from build123d import *

# Parameters (mm, degrees)
F1_DEPTH = 12.7


with BuildPart() as f1:
    # F0 (on Top) → F1 (new body)
    with BuildSketch(Plane.XY):
        with BuildLine():
            Line((0, 52.0365796983), (-20.0025, 52.0365796983))
            Line((-20.0025, 52.0365796983), (-12.633157894, -20.4536858946))
            Line((-12.633157894, -20.4536858946), (-20.0025, -42.7121035755))
            add(Edge.make_bspline(
                [(-20.0025, -42.7121035755), (-21.1866346696, -45.1468080489), (-23.1579199792, -48.7548194432), (-25.0683852323, -64.3099806953), (-16.9383073123, -59.2079587227), (-13.8363149017, -62.2634203017)],
                knots=[0, 0, 0, 0, 0.3090403224, 0.6689788708, 1, 1, 1, 1], degree=3))
            Line((-13.8363149017, -62.2634203017), (0, -62.2634203017))
            Line((0, -62.2634203017), (13.8363149017, -62.2634203017))
            add(Edge.make_bspline(
                [(20.0025, -42.7121035755), (21.1866346696, -45.1468080489), (23.1579199792, -48.7548194432), (25.0683852323, -64.3099806953), (16.9383073123, -59.2079587227), (13.8363149017, -62.2634203017)],
                knots=[0, 0, 0, 0, 0.3090403224, 0.6689788708, 1, 1, 1, 1], degree=3))
            Line((20.0025, -42.7121035755), (12.633157894, -20.4536858946))
            Line((12.633157894, -20.4536858946), (20.0025, 52.0365796983))
            Line((20.0025, 52.0365796983), (0, 52.0365796983))
        make_face()
    extrude(amount=F1_DEPTH)


solid = f1.part
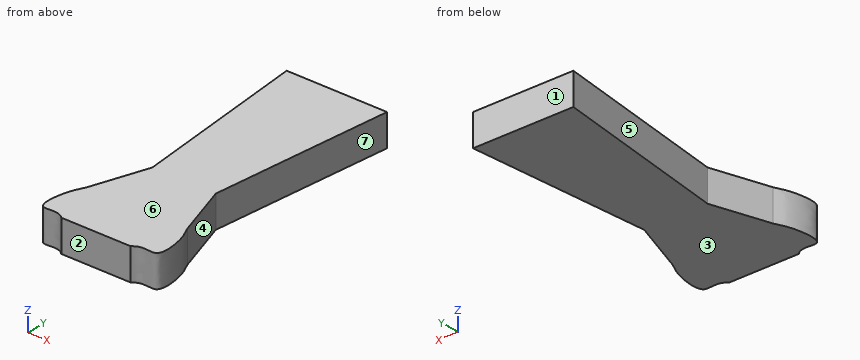
Read the model definition and answer for the solid it produces. Units are mm, in the model's axes. Face numbers are marked on the shaded views. A direction names the side the tool comes from. Coordinates: 2 decimals unless noted, no trailing zeros. Loops run counter-clockwise (first coordinate to the right, second up) from the corner with the lowest first, then second, coordinate; pieces in that order, holes last. Notation, with made-up numbers: (4, 10) -> (32, 10) arc R22 ccw to (32, 46) -> close; hole circle Ø1 at (78.25, 84). An arc over 180 degrees is marked (long way). Answer in a Markdown table with one row per item.
Item 1: Each of these flat-tipped pins is pushed along its axis until it touches: P1, Ø3, axis at y = 30, z = 6.5, coming from the -X side; P2, Ø1.5, axis at y = -28.5, z = 8, coming from the -X side; P3, Ø4, axis at y = 9, z = 4.5, coming from the +X side. Where does it stop, or does it pass through?
Returned:
| item | result |
|---|---|
| P1 | stops at x = -17.91 |
| P2 | stops at x = -15.55 |
| P3 | stops at x = 15.83 |
Item 2: A cutting plane is placed at A-A on y = 5. Determine the outline of the cut face in (x, z), plus the area to 3 significant figures.
Returned:
| item | result |
|---|---|
| outline | (-15.22, 0) -> (15.22, 0) -> (15.22, 12.7) -> (-15.22, 12.7) -> close |
| area | 387 mm^2 |
Item 3: Straight lines are drawn through the part: line 1 along X through (y, z) = (-20.5, 12); line 2 along X through (y, z) = (0, 10.75). For each, find the intervals that lie inside material, in ascending order. Write a range as [from, to].
Returned:
| item | result |
|---|---|
| line 1 | x = [-12.65, 12.65] |
| line 2 | x = [-14.71, 14.71] |
Item 4: For a pull along Y with two mould halves and no side action, classify the marked faces 1, 2, 3 and 4 as released by +Y, released by -Y, zero draft, split by the parting line, or undercut.
Returned:
| item | result |
|---|---|
| face 1 | released by +Y |
| face 2 | released by -Y |
| face 3 | zero draft |
| face 4 | undercut |
Item 5: For the marked faces 5, 6 and 7, determine the directions among +Z, -Z, +X, -X, +Y, -Y from which every point of the face is accessible in a straight line to the end or side of a thin tool.
Returned:
| item | result |
|---|---|
| face 5 | +Z, -Z, -X |
| face 6 | +Z, +X, -X, +Y, -Y |
| face 7 | +Z, -Z, +X |
Item 6: A cutting plane is placed at B-B on y = 22. Determine the outline of the cut face in (x, z), plus the area to 3 significant figures.
Returned:
| item | result |
|---|---|
| outline | (-16.95, 0) -> (16.95, 0) -> (16.95, 12.7) -> (-16.95, 12.7) -> close |
| area | 431 mm^2 |
